Could you check a few things on this model? Use its own coordinates, in mm. A direction names the side the tool comes from. Give positions to 0.01 mm unless a question says otherwise; leave off trailing zeros. Loops run counter-clockwise (first coordinate to the right, second up) from the corner with the lowest first, then second, coordinate; pieces in that order, holes last. Notation, with made-up numbers: (25.5, 80) - (77.5, 80) arc R17 ccw to (77.5, 105) - close; hole circle Ø1 at (47, 62). An arc over 180 degrees is marked (long way). One line per item, written item: value. Start each with the question number.
Q1. I'm going to push flat-ended pins straight in: P1, Ø6, axis at x = -5.38, y = 0, coming from the +Z side; P2, Ø2.5, axis at x = -0.5, z = 2.5, coming from the +Y side; P3, Ø1.5, axis at x = 5.5, z = 4, coming from the +Y side; P4, Ø4, axis at x = -1, z = 3.5, coming from the -Y side. Where does each tip first touch, or does it pass through?
Q2. I want a section at A-A (x = 5.5). Please give me the cut outline in (y, z).
Q3. If I drill on line 1 (Z direction, x = 1, y = 3); line 2 (Z direction, x = 8.75, y = -1.75); line 3 (Y direction, x = -8, z = 0.75), over which ranges is the centre line in solid material (lowest first)? Write a range as from..to.
Q4. I want a section at C-C (x = -5.5). Please give me the cut outline in (y, z), then the cut area to 3 significant figures.
Q5. I want a section at B-B (y = -1). Please give me the cut outline in (x, z), then the cut area to 3 significant figures.
Q6. If we mould it in two halves opening along Y, with no side actions, what happens to faces 6 (the face through (-0.3, -5.7, 0)), 7 (the face through (0.1, -4.5, 0.5)), 8 (the face through (-10.05, 5.57, 2.54))? For each: released by +Y, released by -Y, zero draft, split by the parting line, or undercut.
Q7. For faces 1 (the face through (1, 0, 1)), 2 (the face through (-3, -6, 2)), 3 (the face through (-10.5, 0, 3)), 4 (the face through (-4, -2, 3.5)), 5 (the face through (-3, 6, 2)), which set-ups out of +Z, -Z, +X, -X, +Y, -Y let a thin tool reach every point of the face, with its end or its side?
Q8. I want a section at D-D (z = 5.5). Please give me the cut outline in (x, y).
```python
from build123d import *

# Parameters (mm, degrees)
F1_DEPTH  = 5
F3_DEPTH  = 22.751
F4_R      = 2.25
F5_DEPTH  = 25
F6_R      = 4.1
F6_R_2    = 2.25
F7_DEPTH  = 1.5
F9_DEPTH  = 4
F10_R     = 1.5
F11_R     = 4.85
F12_DEPTH = 5
F13_R     = 1.25
F14_DEPTH = 12.5


# Not quite as in the source:
# - a feature names something its author has since deleted; it is built from what else it names


with BuildPart() as f1:
    # F0 (on Top) → F1 (new body)
    with BuildSketch(Plane.XY):
        with BuildLine():
            Line((-10.5, -6), (2.4076707808, -6))
            ThreePointArc((2.4076707808, -6), (12.25, 0), (2.4076707808, 6))
            Line((2.4076707808, 6), (-10.5, 6))
            Line((-10.5, 6), (-10.5, -6))
        make_face()
    extrude(amount=F1_DEPTH)

    # F2 (on face) → F3 (cut, through all)
    with BuildSketch(Plane(origin=(-10.5, 0, 0), x_dir=(0, -1, 0), z_dir=(-1, 0, 0))):
        Polygon((5, 0), (4, 1), (-4, 1), (-5, 0), align=None)
    extrude(amount=-F3_DEPTH, mode=Mode.SUBTRACT)

    # F4 (on face) → F5 (cut)
    with BuildSketch(Plane.XY.offset(5)):
        with Locations((-5.3849667311, 0)):
            Circle(F4_R)
    extrude(amount=-F5_DEPTH, mode=Mode.SUBTRACT)

    # F6 (on face) → F7 (cut)
    with BuildSketch(Plane.XY.offset(5)):
        with Locations((-5.3849667311, 0)):
            Circle(F6_R)
        with Locations((-5.3849667311, 0)):
            Circle(F6_R_2, mode=Mode.SUBTRACT)
    extrude(amount=-F7_DEPTH, mode=Mode.SUBTRACT)

    # F8 (on face) → F9 (join)
    with BuildSketch(Plane.XY.offset(5)):
        with BuildLine():
            ThreePointArc((2.4076707808, -6), (9.0134938288, -5.7634938288), (12.25, 0))
            ThreePointArc((12.25, 0), (9.0134938288, 5.7634938288), (2.4076707808, 6))
            ThreePointArc((2.4076707808, 6), (-1.25, 0), (2.4076707808, -6))
        make_face()
    extrude(amount=F9_DEPTH)

    # F10
    f10_edges = [f1.edges().sort_by_distance(p)[0] for p in [
        (-10.5, -6, 2.5),
        (-10.5, 6, 2.5),
    ]]
    fillet(f10_edges, radius=F10_R)

    # F11 (on face) → F12 (cut)
    with BuildSketch(Plane.XY.offset(9)):
        with Locations((5.5, 0)):
            Circle(F11_R)
    extrude(amount=-F12_DEPTH, mode=Mode.SUBTRACT)

    # F13 (on Front) → F14 (cut, symmetric)
    with BuildSketch(Plane.XZ):
        with Locations((5.5, 4)):
            Circle(F13_R)
    extrude(amount=F14_DEPTH, both=True, mode=Mode.SUBTRACT)


solid = f1.part
```
Worked answers:
1. P1: stops at z = 3.5
1. P2: stops at y = 6
1. P3: passes through
1. P4: stops at y = -6
2. outline: (-6.75, 0) - (-5, 0) - (-4, 1) - (4, 1) - (5, 0) - (6.75, 0) - (6.75, 2.75) - (-6.75, 2.75) - close; (-6.75, 5.25) - (-4.85, 5.25) - (-4.85, 9) - (-6.75, 9) - close; (4.85, 5.25) - (6.75, 5.25) - (6.75, 9) - (4.85, 9) - close
3. line 1: z = 1..9
3. line 2: z = 1..4
3. line 3: y = -6..-4.25, 4.25..6
4. outline: (-6, 0) - (-5, 0) - (-4, 1) - (-2.25, 1) - (-2.25, 3.5) - (-4.1, 3.5) - (-4.1, 5) - (-6, 5) - close; (2.25, 1) - (4, 1) - (5, 0) - (6, 0) - (6, 5) - (4.1, 5) - (4.1, 3.5) - (2.25, 3.5) - close
4. area: 27.5 mm²
5. outline: (-10.5, 1) - (-7.4, 1) - (-7.4, 3.5) - (-9.36, 3.5) - (-9.36, 5) - (-10.5, 5) - close; (-3.37, 1) - (12.18, 1) - (12.18, 9) - (10.25, 9) - (10.25, 4) - (6.75, 4) arc R1.25 cw to (4.25, 4) - (0.75, 4) - (0.75, 9) - (-1.18, 9) - (-1.18, 5) - (-1.41, 5) - (-1.41, 3.5) - (-3.37, 3.5) - close
5. area: 72.2 mm²
6. face 6: zero draft
6. face 7: undercut
6. face 8: released by +Y
7. face 1: -Z, +X, -X
7. face 2: +Z, -Z, -X, -Y
7. face 3: +Z, -Z, -X, +Y, -Y
7. face 4: +Z
7. face 5: +Z, -Z, -X, +Y
8. outline: circle Ø13.5 at (5.5, 0); hole circle Ø9.7 at (5.5, 0)
